Could you check a few things on this model? Use its own coordinates, in mm. Face numbers are marked on the shaded views. A direction names the side the tool comes from. Give positions to 0.01 mm unless a question says otherwise; leave off trailing zeros. Loops run counter-clockwise (first coordinate to the right, second up) from the corner with the lowest first, then second, coordinate; pieces in that order, holes last. Notation, with made-up numbers: (11.25, 68.5) - (39.25, 68.5) arc R22 cw to (39.25, 102.5) - close; hole circle Ø8 at (60.5, 53). An arc over 180 degrees is marked (long way). Write each question's results on one line, items separated by ' | '. Start each with the question number.
(1) For pin 1 (1.2 mm diameter, centred on x = -6.5, z = 2.5, fed in from -Y); pin 2 (1.2 mm diameter, centred on y = -9.5, z = 2, fed in from +X), each with a flat end and sliding along its axis, tell me the tip position at first contact or that it passes through.
(2) I need wall thicknesses on line 1 (Y direction, x = -5, z = 2.75); line 2 (X direction, y = -17.5, z = 0.95); line 3 (X direction, y = -4, z = 1). Which ranges of each line are inside material? Lowest first, please.
(3) If we mould it in two halves opening along X, with no side actions, what happens to the marked faces 4, 5 and 6? For each: released by +X, released by -X, zero draft, split by the parting line, or undercut.
(4) Suppose I cut it at B-B (z = 1.35). Please give me the cut outline in (x, y).
(5) Suppose I cut it at D-D (y = -14). Please give me the cut outline in (x, z).
(6) Suppose I cut it at C-C (y = 3.75). Please give me the cut outline in (x, z), and give its area (3 significant figures).
(7) On a 3-axis mill with a long thin cutter (end or side, diameter ignored), from which of +Z, -Z, +X, -X, +Y, -Y can I reach the whole of each face in a straight line? I mean the marked faces 1, 2 and 3. Say none if no direction works.
(8) Suppose I cut it at A-A (x = -5). Please give me the cut outline in (y, z), and give its area (3 significant figures).
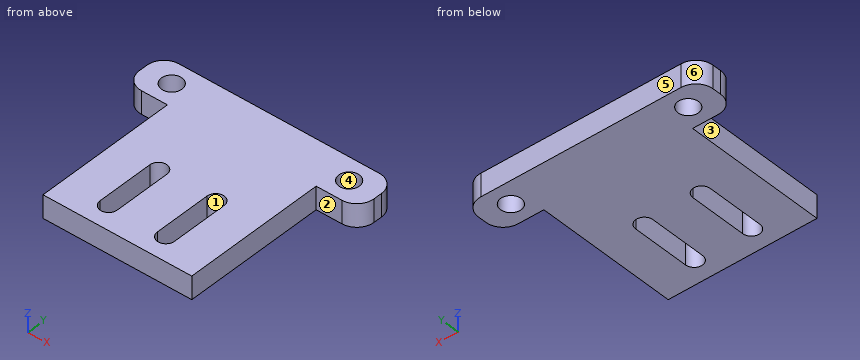
from build123d import *

# Parameters (mm, degrees)
F0_R     = 1.8
F0_W     = 26
F0_H     = 25
F1_DEPTH = 4
F2_R     = 3


# Not quite as in the source:
# - a feature names something its author has since deleted; it is built from what else it names


with BuildPart() as f1:
    # F0 (on Top) → F1 (new body)
    with BuildSketch(Plane.XY):
        Polygon((0, 7.5), (-41, 7.5), (-41, 0), (-33.5, 0), (-7.5, 0), (0, 0), align=None)
        with Locations((-36, 3.75)):
            Circle(F0_R, mode=Mode.SUBTRACT)
        with Locations((-5, 3.75)):
            Circle(F0_R, mode=Mode.SUBTRACT)
        with Locations((-20.5, -12.5)):
            Rectangle(F0_W, F0_H)
        with BuildLine():
            Line((-27, -21), (-27, -11))
            ThreePointArc((-27, -11), (-25.5, -9.5), (-24, -11))
            Line((-24, -11), (-24, -21))
            ThreePointArc((-24, -21), (-25.5, -22.5), (-27, -21))
        make_face(mode=Mode.SUBTRACT)
        with BuildLine():
            Line((-17, -21), (-17, -11))
            ThreePointArc((-17, -11), (-15.5, -9.5), (-14, -11))
            Line((-14, -11), (-14, -21))
            ThreePointArc((-14, -21), (-15.5, -22.5), (-17, -21))
        make_face(mode=Mode.SUBTRACT)
    extrude(amount=F1_DEPTH)

    # F2
    f2_edges = [f1.edges().sort_by_distance(p)[0] for p in [
        (0, 0, 2),
        (0, 7.5, 2),
        (-41, 0, 2),
        (-41, 7.5, 2),
    ]]
    fillet(f2_edges, radius=F2_R)


solid = f1.part
Output values:
1) pin 1: y = 0 | pin 2: x = -7.5
2) line 1: 0 to 1.95, 5.55 to 7.5 | line 2: -33.5 to -27, -24 to -17, -14 to -7.5 | line 3: -33.5 to -7.5
3) face 4: undercut | face 5: zero draft | face 6: released by -X
4) outline: (-41, 3) arc R3 ccw to (-38, 0) - (-33.5, 0) - (-33.5, -25) - (-7.5, -25) - (-7.5, 0) - (-3, 0) arc R3 ccw to (0, 3) - (0, 4.5) arc R3 ccw to (-3, 7.5) - (-38, 7.5) arc R3 ccw to (-41, 4.5) - close; hole circle Ø3.6 at (-36, 3.75); hole (-27, -21) arc R1.5 ccw to (-24, -21) - (-24, -11) arc R1.5 ccw to (-27, -11) - close; hole (-17, -21) arc R1.5 ccw to (-14, -21) - (-14, -11) arc R1.5 ccw to (-17, -11) - close; hole circle Ø3.6 at (-5, 3.75)
5) outline: (-33.5, 0) - (-27, 0) - (-27, 4) - (-33.5, 4) - close; (-24, 0) - (-17, 0) - (-17, 4) - (-24, 4) - close; (-14, 0) - (-7.5, 0) - (-7.5, 4) - (-14, 4) - close
6) outline: (-41, 0) - (-37.8, 0) - (-37.8, 4) - (-41, 4) - close; (-34.2, 0) - (-6.8, 0) - (-6.8, 4) - (-34.2, 4) - close; (-3.2, 0) - (0, 0) - (0, 4) - (-3.2, 4) - close | area: 135 mm2
7) face 1: +Z, -Z | face 2: +Z, -Z, +X, -Y | face 3: +Z, -Z, -X, -Y
8) outline: (0, 0) - (1.95, 0) - (1.95, 4) - (0, 4) - close; (5.55, 0) - (7.5, 0) - (7.5, 4) - (5.55, 4) - close | area: 15.6 mm2
